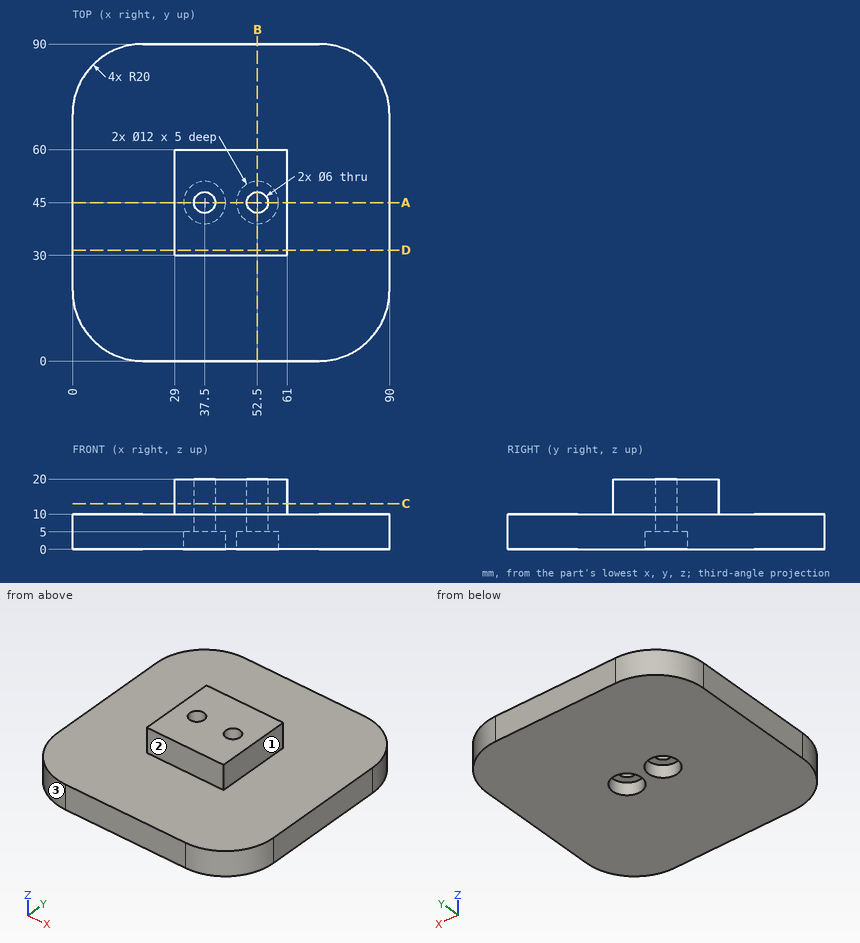
Source: three-view drawing plus pictorial views. Frame: mm from the lowest corner of the part. A direction names the side the tool comes from. Round coordinates to 2 decimals unless told otherwise and drop trailing zeros. Loops run counter-clockwise (first coordinate to the right, second up) from the corner with the lowest first, then second, coordinate; pieces in that order, holes last.
Q1. Section A-A, the plane y = 45. Return loops of the section in (x, z).
Q2. Section C-C, the plane z = 13. Return loops of the section in (x, y).
Q3. Access query for the marked faces 1, 2 and 3. Directions: +Z, -Z, +X, -X, +Y, -Y. A direction counts if a zero-diameter tool reaches every point of the face in a straight line with its end or side. Return the directions, or none.
Q4. First-contact query: P1, Ø6, axis at x = 53, y = 43.5, coming from the -Z side; P2, Ø11, axis at y = 42, z = 16, coming from the +X side; P3, Ø6, axis at x = 57.5, y = 22.5, coming from the +Z side; P4, Ø6, axis at y = 74.5, z = 15.5, coming from the -X side. Flat tips, straight axial feed; report the tip coordinate or a pass-through.
Q5. Ray query, line 1 (Y direction, x = 37.5, z = 1.1); line 2 (Z direction, x = 63, y = 70.5); line 3 (Y direction, x = 52.5, z = 15). Return the intervals inside material, ascending.
Q6. Section B-B, the plane x = 52.5. Return loops of the section in (y, z), plus the area to 3 significant figures.
Q7. Section D-D, the plane y = 31.5. Return loops of the section in (x, z), plus the area to 3 significant figures.
Solutions:
1. outline: (0, 0) - (31.5, 0) - (31.5, 5) - (34.5, 5) - (34.5, 20) - (29, 20) - (29, 10) - (0, 10) - close; (40.5, 5) - (43.5, 5) - (43.5, 0) - (46.5, 0) - (46.5, 5) - (49.5, 5) - (49.5, 20) - (40.5, 20) - close; (55.5, 5) - (58.5, 5) - (58.5, 0) - (90, 0) - (90, 10) - (61, 10) - (61, 20) - (55.5, 20) - close
2. outline: (29, 30) - (61, 30) - (61, 60) - (29, 60) - close; hole circle Ø6 at (37.5, 45); hole circle Ø6 at (52.5, 45)
3. face 1: +Z, +X, +Y, -Y
3. face 2: +Z, +X, -X, -Y
3. face 3: +Z, -Z, -X, -Y
4. P1: stops at z = 5
4. P2: stops at x = 61
4. P3: stops at z = 10
4. P4: passes through
5. line 1: y = 0 to 39, 51 to 90
5. line 2: z = 0 to 10
5. line 3: y = 30 to 42, 48 to 60
6. outline: (0, 0) - (39, 0) - (39, 5) - (42, 5) - (42, 20) - (30, 20) - (30, 10) - (0, 10) - close; (48, 5) - (51, 5) - (51, 0) - (90, 0) - (90, 10) - (60, 10) - (60, 20) - (48, 20) - close
6. area: 1,050 mm2
7. outline: (0, 0) - (90, 0) - (90, 10) - (61, 10) - (61, 20) - (29, 20) - (29, 10) - (0, 10) - close
7. area: 1,220 mm2
